from build123d import *

# Parameters (mm, degrees)
CROQUIS1_R              = 82.42
SALIENTE_EXTRUIR1_DEPTH = 5
CROQUIS2_R              = 100
SALIENTE_EXTRUIR2_DEPTH = 5
CROQUIS3_R              = 2.5
CORTAR_EXTRUIR1_DEPTH   = 10
CROQUIS4_R              = 2.5
CORTAR_EXTRUIR2_DEPTH   = 10


with BuildPart() as part:
    # Croquis1 → Saliente-Extruir1 (new body)
    with BuildSketch(Plane.XY):
        Circle(CROQUIS1_R)
    extrude(amount=SALIENTE_EXTRUIR1_DEPTH)

    # Croquis2 → Saliente-Extruir2 (add)
    with BuildSketch(Plane.XY.offset(5)):
        Circle(CROQUIS2_R)
    extrude(amount=-SALIENTE_EXTRUIR2_DEPTH)

    # Croquis3 → Cortar-Extruir1 (cut)
    with BuildSketch(Plane.XY.offset(5)):
        with Locations((-37, -80.903175403)):
            Circle(CROQUIS3_R)
        with Locations((37, -80.903175403)):
            Circle(CROQUIS3_R)
        with Locations((-37, -41.303175403)):
            Circle(CROQUIS3_R)
        with Locations((37, -41.303175403)):
            Circle(CROQUIS3_R)
    extrude(amount=-CORTAR_EXTRUIR1_DEPTH, mode=Mode.SUBTRACT)

    # Croquis4 → Cortar-Extruir2 (cut)
    with BuildSketch(Plane.XY.offset(5)):
        with Locations((-37, -41.303175403)):
            Circle(CROQUIS4_R)
        with Locations((-37, 39.446824597)):
            Circle(CROQUIS4_R)
        with Locations((-37, -80.903175403)):
            Circle(CROQUIS4_R)
        with Locations((-37, 79.046824597)):
            Circle(CROQUIS4_R)
        with Locations((37, -41.303175403)):
            Circle(CROQUIS4_R)
        with Locations((37, 79.046824597)):
            Circle(CROQUIS4_R)
        with Locations((37, 39.446824597)):
            Circle(CROQUIS4_R)
    extrude(amount=-CORTAR_EXTRUIR2_DEPTH, mode=Mode.SUBTRACT)


solid = part.part
Build history of the part. All positions in model axes, mm. Round coordinates to 2 decimals unless told otherwise and drop trailing zeros. Loops run counter-clockwise (first coordinate to the right, second up) from the corner with the lowest first, then second, coordinate; pieces in that order, holes last. Notation, with made-up numbers: (-26, 18.5) -> (-8, 18.5) arc R21 ccw to (-8, 26.5) -> close; hole circle Ø8 at (-36.5, -36). An arc over 180 degrees is marked (long way). One line per item, written item: value. Start each with the question number.
Q1. Cut at C-C on y = 49. List the corners of the cut face in (x, z), plus the area to 3 significant figures.
Q2. Probe line 1 along X through (y, z) = (-41.5, 1.45); line 2 along Y through (x, z) = (-37, 3.15); line 3 along Y through (x, z) = (-35, 3.9). List the from-to ranges inside material, lowest first.
Q3. Cut at A-A on x = 37. List the corners of the cut face in (y, z), plus the area to 3 significant figures.
Q4. Two-plate mould, pull along Y, no slides. Class faces 1 (the face through (-1, 1, 5)), 2 (the face through (-35.846, -83.121, 2.535)), 3 (the face through (95.38, 30.04, 2.54)): released by +Y, released by -Y, zero draft, split by the parting line, or undercut.
Q5. Cut at B-B on z = 3.1. Count the separate pieces of the cut face and the enclosed holes in it, plus the area to 3 significant figures.
Q6. Cut at D-D on x = -26. List the corners of the cut face in (y, z).
Q7. Drop flat-ended pins along their axis: pin 1 Ø3 at (x, y) = (-64.5, 32) entering from -Z; pin 2 Ø3 at (x, y) = (37, 79.05) entering from -Z; pin 3 Ø1.5 at (x, z) = (-10.5, 4) entering from -Y; pin 4 Ø1 at (x, z) = (40, 0.5) entering from +Y. Give the stop position or say it passes through.
Computed:
1. outline: (-87.17, 0) -> (87.17, 0) -> (87.17, 5) -> (-87.17, 5) -> close
1. area: 872 mm²
2. line 1: -90.98 to -39.49, -34.51 to 34.51, 39.49 to 90.98
2. line 2: -92.9 to -83.4, -78.4 to -43.8, -38.8 to 36.95, 41.95 to 76.55, 81.55 to 92.9
2. line 3: -93.67 to -82.4, -79.4 to -42.8, -39.8 to 37.95, 40.95 to 77.55, 80.55 to 93.67
3. outline: (-92.9, 0) -> (-83.4, 0) -> (-83.4, 5) -> (-92.9, 5) -> close; (-78.4, 0) -> (-43.8, 0) -> (-43.8, 5) -> (-78.4, 5) -> close; (-38.8, 0) -> (36.95, 0) -> (36.95, 5) -> (-38.8, 5) -> close; (41.95, 0) -> (76.55, 0) -> (76.55, 5) -> (41.95, 5) -> close; (81.55, 0) -> (92.9, 0) -> (92.9, 5) -> (81.55, 5) -> close
3. area: 829 mm²
4. face 1: zero draft
4. face 2: undercut
4. face 3: split by the parting line
5. separate pieces: 1
5. enclosed holes: 8
5. area: 31,300 mm²
6. outline: (-96.56, 0) -> (96.56, 0) -> (96.56, 5) -> (-96.56, 5) -> close
7. pin 1: z = 0
7. pin 2: through
7. pin 3: y = -99.52
7. pin 4: y = 91.87
